Geometry check sheet. Reference: drawing and pictorial views, mm from the part's lowest x, y, z. A direction names the side the tool comes from. Give positions to 0.01 mm unless a question says otherwise; leave off trailing zeros. Write each loop counter-clockwise with the first axis right and the second up, starting at its lowest first coordinate (ties: lowest second). Pieces come first, ordered by that corner, then holes. Notation, with made-up numbers: (-28, 49.5) - (-8, 49.5) arc R35 ccw to (-8, 88.5) - close; hole circle Ø6 at (15, -32.75). An arc over 180 degrees is marked (long way). Put each result on its own line as item: value.
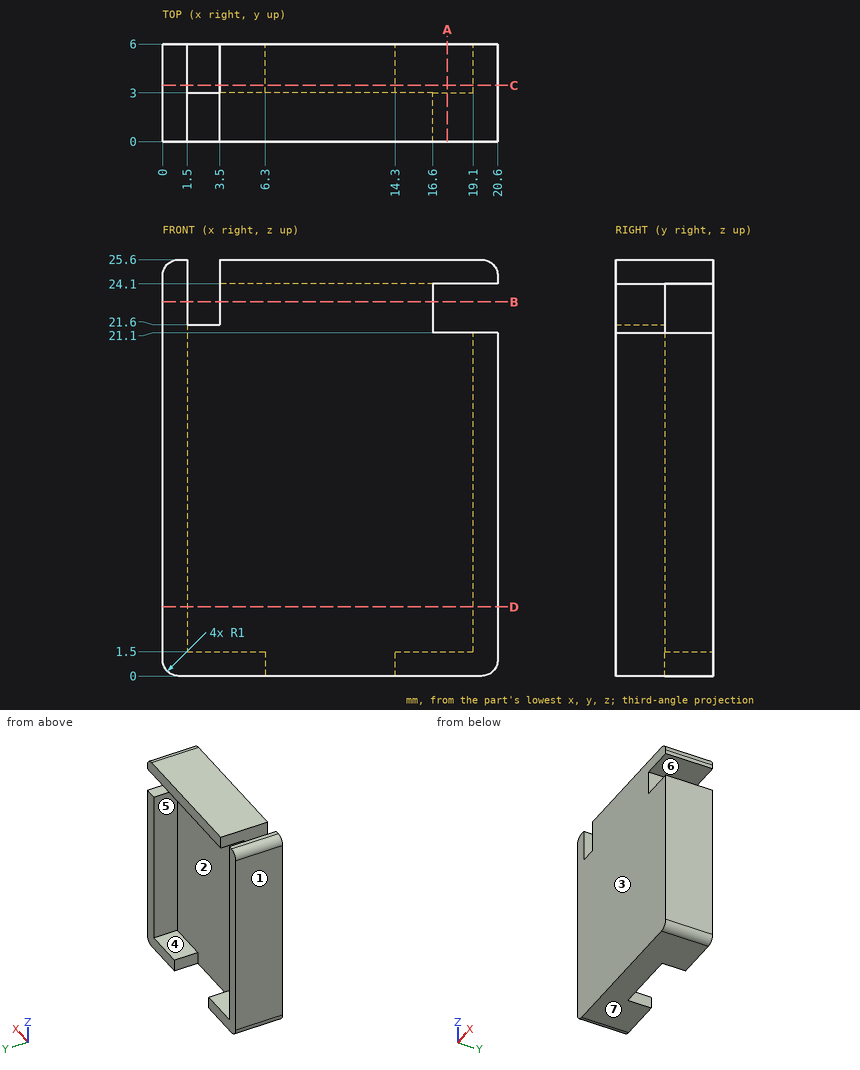
Q1. Release check for a two-part mould opening along X. For the marked faces 1, 2, 3 and 4 record: released by +X, released by -X, zero draft, split by the parting line, or undercut.
Answers follow:
face 1: released by -X
face 2: undercut
face 3: zero draft
face 4: undercut
Q2. Section check B-B, the plane z = 23. Record the cut outline in (x, y).
Answers follow:
outline: (0, 0) - (1.5, 0) - (1.5, 6) - (0, 6) - close; (3.5, 0) - (16.6, 0) - (16.6, 3) - (3.5, 3) - close
Q3. Go/stop test with flat-tipped pins: pin 1 Ø5.5 at (x, z) = (9, 15.5) entering from +Y; pin 2 Ø0.9 at (x, y) = (3, 4.5) entering from +Z; pin 3 Ø0.6 at (x, y) = (2, 1.5) entering from +Z. Record where each tip stops, or that it passes through.
Answers follow:
pin 1: stops at y = 3
pin 2: stops at z = 1.5
pin 3: stops at z = 21.6
Q4. Section check C-C, the plane y = 3.45. Record the cut outline in (x, z).
Answers follow:
outline: (0, 1) arc R1 ccw to (1, 0) - (6.3, 0) - (6.3, 1.5) - (1.5, 1.5) - (1.5, 25.6) - (1, 25.6) arc R1 ccw to (0, 24.6) - close; (3.5, 24.1) - (20.6, 24.1) - (20.6, 24.6) arc R1 ccw to (19.6, 25.6) - (3.5, 25.6) - close; (14.3, 0) - (19.6, 0) arc R1 ccw to (20.6, 1) - (20.6, 21.1) - (19.1, 21.1) - (19.1, 1.5) - (14.3, 1.5) - close
Q5. Set-up check for the marked faces 5, 6 and 7: record each of +Z, -Z, +X, -X, +Y, -Y from which the full face is reachable in a straight line by a thin tool's end or side.
Answers follow:
face 5: +Y
face 6: +X, +Y
face 7: -Z, +X, -X, +Y, -Y
Q6. Section check A-A, the plane x = 17.5. Record the cut outline in (y, z), plus the area to 3 significant figures.
Answers follow:
outline: (0, 0) - (6, 0) - (6, 1.5) - (3, 1.5) - (3, 21.1) - (0, 21.1) - close; (0, 24.1) - (6, 24.1) - (6, 25.6) - (0, 25.6) - close
area: 76.8 mm2
Q7. Section check D-D, the plane z = 4.25. Record the cut outline in (x, y).
Answers follow:
outline: (0, 0) - (20.6, 0) - (20.6, 6) - (19.1, 6) - (19.1, 3) - (1.5, 3) - (1.5, 6) - (0, 6) - close
Q8. Scan lines: line 1 along X through (y, z) = (5.35, 18.75); line 2 along Z through (x, y) = (18.5, 5.55); line 3 along Z through (x, y) = (17, 2.95). Record each from-to range of solid material in increasing order.
Answers follow:
line 1: x = 0 to 1.5, 19.1 to 20.6
line 2: z = 0 to 1.5, 24.1 to 25.6
line 3: z = 0 to 21.1, 24.1 to 25.6
